from build123d import *

# Parameters (mm, degrees)
EXTRUDE_1_DEPTH = 90
EXTRUDE_START   = -3
EXTRUDE_2_DEPTH = 3


with BuildPart() as part:
    # 草图2 → 旋转1 (revolve)
    with BuildSketch(Plane.XY, mode=Mode.PRIVATE) as revolve_1_sk:
        with BuildLine():
            Line((20, -224.411230387), (20, -214.411230387))
            Line((20, -214.411230387), (17.5, -214.411230387))
            Line((17.5, -214.411230387), (17.5, -209.411230387))
            Line((17.5, -209.411230387), (20, -209.411230387))
            Line((20, -209.411230387), (20, -204.411230387))
            Line((20, -204.411230387), (17.5, -204.411230387))
            Line((17.5, -204.411230387), (17.5, -199.411230387))
            Line((17.5, -199.411230387), (20, -199.411230387))
            Line((20, -199.411230387), (20, -194.411230387))
            Line((20, -194.411230387), (17.5, -194.411230387))
            Line((17.5, -194.411230387), (17.5, -189.411230387))
            Line((17.5, -189.411230387), (20, -189.411230387))
            Line((20, -189.411230387), (20, -174.411230387))
            ThreePointArc((20, -174.411230387), (20.676631798, -170.795320354), (22.614961073, -167.668738262))
            Line((22.614961073, -167.668738262), (35.258140309, -153.820687856))
            ThreePointArc((35.258140309, -153.820687856), (37.196469585, -150.694105764), (37.873101383, -147.078195731))
            Line((37.873101383, -147.078195731), (37.873101383, -54.411230387))
            Line((37.873101383, -54.411230387), (35.873101383, -54.411230387))
            Line((35.873101383, -54.411230387), (35.873101383, -129.659355933))
            ThreePointArc((35.873101383, -129.659355933), (31.874010536, -149.253139566), (20.5164471, -165.712630368))
            Line((20.5164471, -165.712630368), (18.571330856, -167.581679311))
            ThreePointArc((18.571330856, -167.581679311), (16.299818169, -170.873577472), (15.5, -174.792334198))
            Line((15.5, -174.792334198), (15.5, -224.411230387))
            Line((15.5, -224.411230387), (20, -224.411230387))
        make_face()
    revolve(revolve_1_sk.sketch.rotate(Axis((0, -59.896764436, 0), (0, -1, 0)), 180), axis=Axis((0, -59.896764436, 0), (0, -1, 0)))

    # 草图4 → 凸台-拉伸1 (add)
    with BuildSketch(Plane(origin=(0, -54.411230387, 0), x_dir=(1, 0, 0), z_dir=(0, 1, 0))):
        with BuildLine():
            ThreePointArc((-35.873101383, -12.144645138), (-37.369756581, -6.154112558), (-37.873101383, 0))
            Line((-37.873101383, 0), (-37.873101383, -23.873101383))
            ThreePointArc((-37.873101383, -23.873101383), (-40.802033571, -30.944169195), (-47.873101383, -33.873101383))
            Line((-47.873101383, -33.873101383), (-55, -33.873101383))
            Line((-55, -33.873101383), (-55, -37.873101383))
            Line((-55, -37.873101383), (0, -37.873101383))
            ThreePointArc((0, -37.873101383), (-8.703229445, -36.859538868), (-16.940626053, -33.873101383))
            Line((-16.940626053, -33.873101383), (-25.873101383, -33.873101383))
            ThreePointArc((-25.873101383, -33.873101383), (-32.944169195, -30.944169195), (-35.873101383, -23.873101383))
            Line((-35.873101383, -23.873101383), (-35.873101383, -12.144645138))
        make_face()
        with BuildLine():
            Line((37.873101383, -23.873101383), (37.873101383, 0))
            ThreePointArc((37.873101383, 0), (37.369756581, -6.154112558), (35.873101383, -12.144645138))
            Line((35.873101383, -12.144645138), (35.873101383, -23.873101383))
            ThreePointArc((35.873101383, -23.873101383), (32.944169195, -30.944169195), (25.873101383, -33.873101383))
            Line((25.873101383, -33.873101383), (16.940626053, -33.873101383))
            ThreePointArc((16.940626053, -33.873101383), (8.703229445, -36.859538868), (0, -37.873101383))
            Line((0, -37.873101383), (55, -37.873101383))
            Line((55, -37.873101383), (55, -33.873101383))
            Line((55, -33.873101383), (47.873101383, -33.873101383))
            ThreePointArc((47.873101383, -33.873101383), (40.802033571, -30.944169195), (37.873101383, -23.873101383))
        make_face()
        with BuildLine():
            ThreePointArc((0, -35.873101383), (-5.98941578, -35.369567448), (-11.810690307, -33.873101383))
            Line((-11.810690307, -33.873101383), (-16.940626053, -33.873101383))
            ThreePointArc((-16.940626053, -33.873101383), (-8.703229445, -36.859538868), (0, -37.873101383))
            Line((0, -37.873101383), (0, -35.873101383))
        make_face()
        with BuildLine():
            Line((16.940626053, -33.873101383), (11.810690307, -33.873101383))
            ThreePointArc((11.810690307, -33.873101383), (5.98941578, -35.369567448), (0, -35.873101383))
            Line((0, -35.873101383), (0, -37.873101383))
            ThreePointArc((0, -37.873101383), (8.703229445, -36.859538868), (16.940626053, -33.873101383))
        make_face()
    extrude(amount=-EXTRUDE_1_DEPTH)

    # 草图3 → 凸台-拉伸2 (add)
    with BuildSketch(Plane(origin=(0, -54.411230387, 0), x_dir=(1, 0, 0), z_dir=(0, 1, 0)).offset(EXTRUDE_START)):
        with BuildLine():
            ThreePointArc((35.873101383, 0), (25.36611325, 25.36611325), (0, 35.873101383))
            Line((0, 35.873101383), (0, 2.25))
            ThreePointArc((0, 2.25), (1.590990258, 1.590990258), (2.25, 0))
            ThreePointArc((2.25, 0), (1.590990258, -1.590990258), (0, -2.25))
            Line((0, -2.25), (0, -35.873101383))
            ThreePointArc((0, -35.873101383), (25.36611325, -25.36611325), (35.873101383, 0))
        make_face()
        with BuildLine():
            Line((0, 2.25), (0, 35.873101383))
            ThreePointArc((0, 35.873101383), (-35.873101383, 0), (0, -35.873101383))
            Line((0, -35.873101383), (0, -2.25))
            ThreePointArc((0, -2.25), (-2.25, 0), (0, 2.25))
        make_face()
        with BuildLine():
            ThreePointArc((37.873101383, 0), (26.780326812, 26.780326812), (0, 37.873101383))
            Line((0, 37.873101383), (0, 35.873101383))
            ThreePointArc((0, 35.873101383), (25.36611325, 25.36611325), (35.873101383, 0))
            ThreePointArc((35.873101383, 0), (25.36611325, -25.36611325), (0, -35.873101383))
            Line((0, -35.873101383), (0, -37.873101383))
            ThreePointArc((0, -37.873101383), (26.780326812, -26.780326812), (37.873101383, 0))
        make_face()
        with BuildLine():
            Line((0, 35.873101383), (0, 37.873101383))
            ThreePointArc((0, 37.873101383), (-37.873101383, 0), (0, -37.873101383))
            Line((0, -37.873101383), (0, -35.873101383))
            ThreePointArc((0, -35.873101383), (-35.873101383, 0), (0, 35.873101383))
        make_face()
    extrude(amount=EXTRUDE_2_DEPTH)


solid = part.part
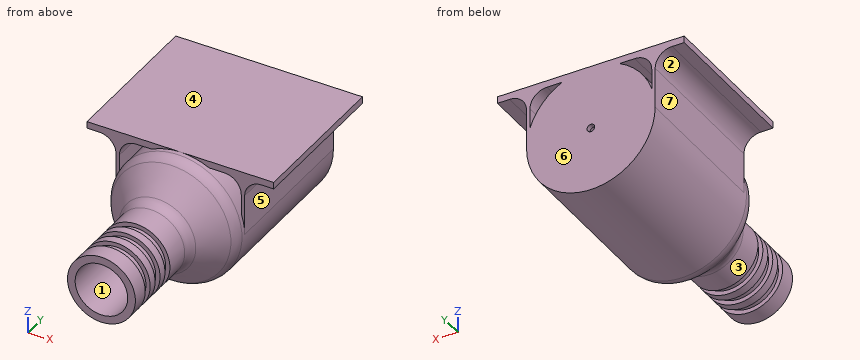
Design review of the part built by this model. Coordinates are the model's own, in mm. Face numbers are marked on the shaded views. A direction names the side the tool comes from. Give positions to 0.01 mm unless a question says otherwise; leave off trailing zeros. Order: outer loops, then holes, each group sorted by start corner. A loop starts at its lowest first (then second) coordinate and runs counter-clockwise, first axis right, second up. Notation, with made-up numbers: (8.25, 4.25) - (40.25, 4.25) arc R30 ccw to (40.25, 30.25) - close; hole circle Ø8 at (0, 19.25). An arc over 180 degrees is marked (long way). Use CSV: the item, a comma, the result in double quotes. Start each with the question number.
Q1. Take a section at A-A (y = -118.5). State the section outline as (x, z) points.
Q2. For line 1 (Y direction, x = 16.5, z = -8.5); line 2 (Z direction, x = 0, y = -208); line 3 (Z direction, x = 0, y = -191), list the stretches that pass through material, from the lowest coordinate up.
Q3. Machinability: for the marked faces 5, 6 and 7, which of the approach directions +Z, -Z, +X, -X, +Y, -Y give a long, thin tool a straight path to every point of the face, cutting with its end or side? Answer none if there is none.
Q4. Draft analysis for pull direction Z (two halves, no side actions). For the marked faces 1, 2, 3 and 4, state which applies: pulls with the +Z half, pulls with the -Z half, needs draft (parallel to the pull), parting line crosses it, or undercut.
Q5. For P1, Ø19, axis at y = -100, z = 11.5, coming from the -X side; P2, Ø10, axis at y = -173.5, z = 1.5, coming from the -X side; P3, Ø12, axis at x = 8.5, z = -0.5, coming from the -Y side, all flat-tipped, find the tip position at first contact; note any pin that passes through.
Calculated:
1,outline,"(-55, 33.87) - (-47.87, 33.87) arc R10 cw to (-37.87, 23.87) - (-37.87, 0) arc R37.87 ccw to (37.87, 0) - (37.87, 23.87) arc R10 cw to (47.87, 33.87) - (55, 33.87) - (55, 37.87) - (-55, 37.87) - close; hole circle Ø71.75 at (0, 0); hole (-35.87, 12.14) arc R37.87 cw to (-16.94, 33.87) - (-25.87, 33.87) arc R10 ccw to (-35.87, 23.87) - close; hole (16.94, 33.87) arc R37.87 cw to (35.87, 12.14) - (35.87, 23.87) arc R10 ccw to (25.87, 33.87) - close"
2,line 1,"y = -224.41 to -214.41, -209.41 to -204.41, -199.41 to -194.41, -189.41 to -167.59, -57.41 to -54.41"
2,line 2,"z = -20 to -15.5, 15.5 to 20"
2,line 3,"z = -17.5 to -15.5, 15.5 to 17.5"
3,face 5,"-Z, +X, +Y, -Y"
3,face 6,"+Z, -Z, +X, -X, +Y"
3,face 7,"-Z, -X, +Y, -Y"
4,face 1,"undercut"
4,face 2,"pulls with the -Z half"
4,face 3,"parting line crosses it"
4,face 4,"pulls with the +Z half"
5,P1,"stops at x = -37.87"
5,P2,"stops at x = -21.9"
5,P3,"stops at y = -57.41"
